Could you check a few things on this model? Use its own coordinates, in mm. A direction names the side the tool comes from. Give positions to 0.01 mm unless a question says otherwise; leave off trailing zeros. Order: outer loops, then holes, each group sorted by start corner. A loop starts at its lowest first (then second) coordinate and runs counter-clockwise, first axis right, second up. Notation, with made-up numbers: (88.25, -26.5) - (97.25, -26.5) arc R21 ccw to (97.25, -13.5) - close; hole circle Ø11 at (47.25, -2.5). An arc over 180 degrees is marked (long way). Put each result on its own line as item: value.
from build123d import *

# Parameters (mm, degrees)
F1_DEPTH        = 25
F3_D            = 13.2
F3_CBORE_D      = 19.25
F3_CBORE_DEPTH  = 0
F4_W            = 24.2927655578
F4_H            = 50
F5_DEPTH        = 60
F7_D            = 13.2
F7_CBORE_D      = 19.25
F7_CBORE_DEPTH  = 0
F9_R            = 15
F10_DEPTH       = 52
F12_D           = 13.2
F12_CBORE_D     = 19.25
F12_CBORE_DEPTH = 0
F13_W           = 29.7532882541
F13_H           = 56.5460538492
F14_DEPTH       = 50


with BuildPart() as f1:
    # F0 (on Front) → F1 (new body)
    with BuildSketch(Plane.XZ):
        with BuildLine():
            Line((-25, -40), (25, -40))
            Line((25, -40), (25, 40))
            ThreePointArc((25, 40), (10.5, 25.5), (-4, 40))
            Line((-4, 40), (-25, 40))
            Line((-25, 40), (-25, -40))
        make_face()
        with BuildLine():
            ThreePointArc((-4, 40), (10.5, 25.5), (25, 40))
            Line((25, 40), (-4, 40))
        make_face()
        with BuildLine():
            Line((-4, 40), (25, 40))
            ThreePointArc((25, 40), (10.5, 54.5), (-4, 40))
        make_face()
    extrude(amount=F1_DEPTH)

    # F3 (through all)
    with Locations(Plane(origin=(0, 0, 0), x_dir=(-1, 0, 0), z_dir=(0, 1, 0))):
        with Locations((-10.5, 40)):
            CounterBoreHole(F3_D / 2, F3_CBORE_D / 2, F3_CBORE_DEPTH)

    # F4 (on Right) → F5 (cut)
    with BuildSketch(Plane.YZ):
        with Locations((-37.1463827789, -15)):
            Rectangle(F4_W, F4_H)
    extrude(amount=F5_DEPTH, mode=Mode.SUBTRACT)

    # F7 (through all)
    with Locations(Plane.XY.offset(40)):
        with Locations((-14.5, -12.5)):
            CounterBoreHole(F7_D / 2, F7_CBORE_D / 2, F7_CBORE_DEPTH)

    # F9 (on face) → F10 (join)
    with BuildSketch(Plane(origin=(0, -36.0705080757, -20.8253175473), x_dir=(-1, 0, 0), z_dir=(0, 0.8660254038, 0.5))):
        with Locations((-25, -22.1410161514)):
            Circle(F9_R)
    extrude(amount=F10_DEPTH)

    # F12 (through all)
    with Locations(Plane(origin=(0, -36.0705080757, -20.8253175473), x_dir=(1, 0, 0), z_dir=(0, -0.8660254038, -0.5))):
        with Locations((25, -22.1410161514)):
            CounterBoreHole(F12_D / 2, F12_CBORE_D / 2, F12_CBORE_DEPTH)

    # F13 (on Right) → F14 (cut)
    with BuildSketch(Plane.YZ):
        with Locations((14.8766441271, -15.394736547)):
            Rectangle(F13_W, F13_H)
    extrude(amount=F14_DEPTH, mode=Mode.SUBTRACT)


solid = f1.part
1) Which directions (+Z, -Z, +X, -X, +Y, -Y) give clear straight access to the entire face, cutting with the end or side of a thin tool? Please do faces 1 (the flat face through (0, -25, 8)), 2 (the cylindrical face through (5.262, -12.675, 35.984)).
Filled in:
face 1: +Z, -X, -Y
face 2: +Y, -Y
2) We'd pull the mould along X, two halves only. Please class faces 3 (the cylindrical face through (-9.262, -16.516, -0.56)), 4 (the cylindrical face through (25.86, -17.04, -27.85)), 5 (the flat face through (-7, -12, 40)), 6 (the flat face through (25, -12, 15)): pulls with the +X half, pulls with the -X half, needs draft (parallel to the pull), parting line crosses it, or undercut.
Filled in:
face 3: undercut
face 4: undercut
face 5: needs draft
face 6: pulls with the +X half
3) I'm going to push flat-ended pins straight in: pin 1 (7.5 mm diameter, centred on y = -9, z = 13, fed in from +X); pin 2 (17 mm diameter, centred on x = -18, y = -7, fed in from +Z); pin 3 (1.5 mm diameter, centred on x = 6.5, y = -6, fed in from +Z); pin 4 (8 mm diameter, centred on x = -14.5, y = -12.5, fed in from -Z). Where does each tip first touch, or does it pass through?
Filled in:
pin 1: stops at x = 25
pin 2: stops at z = 40
pin 3: stops at z = 54.13
pin 4: passes through
4) Suppose I cut it at A-A, the plane z = 38.5. List the corners of the cut face in (x, y) for me, and give its area (3 significant figures).
Filled in:
outline: (-25, -25) - (4.07, -25) - (4.07, 0) - (-25, 0) - close; (16.93, -25) - (25, -25) - (25, 0) - (16.93, 0) - close; hole circle Ø13.2 at (-14.5, -12.5)
area: 792 mm^2
5) Suppose I cut it at D-D, the plane y = -12.5. State how many separate pieces and enclosed holes the cut face has, and give its area (3 significant figures).
Filled in:
separate pieces: 2
enclosed holes: 2
area: 3,490 mm^2
6) If I drill on line 1 (Y direction, x = 19, z = 26.5); line 2 (Y direction, x = -15, z = -4); line 3 (Z direction, x = 10, y = -18), over which ranges is the centre line in solid material (lowest first)? Write a range as [from, to].
Filled in:
line 1: y = [-25, 0]
line 2: y = [-25, -19.08], [-5.92, 0]
line 3: z = [-40, 33.42], [46.58, 54.49]
7) Suppose I cut it at B-B, the plane x = -10. List the corners of the cut face in (y, z) for me.
Filled in:
outline: (-25, -40) - (-17.33, -40) - (-17.33, 40) - (-25, 40) - close; (-7.67, -40) - (0, -40) - (0, 40) - (-7.67, 40) - close
8) Suppose I cut it at C-C, the plane z = 3.5. List the corners of the cut face in (x, y) for me, and give its area (3 significant figures).
Filled in:
outline: (-25, -25) - (25, -25) - (25, 0) - (-25, 0) - close; hole circle Ø13.2 at (-14.5, -12.5)
area: 1,110 mm^2
